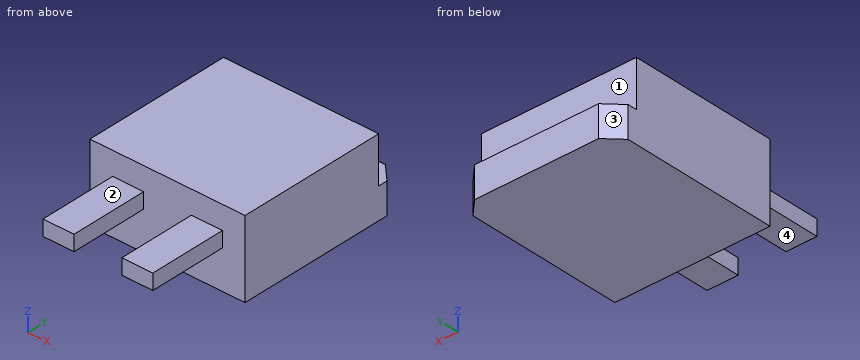
```python
from build123d import *

# Parameters (mm, degrees)
F0_W     = 10
F0_H     = 11.2
F1_DEPTH = 5
F2_W     = 10
F2_H     = 1.6
F3_DEPTH = 3
F4_SIZE  = 1
F5_W     = 2
F5_H     = 1
F6_DEPTH = 5


with BuildPart() as f1:
    # F0 (on Top) → F1 (new body)
    with BuildSketch(Plane.XY):
        with Locations((2.165886, -0.248423)):
            Rectangle(F0_W, F0_H)
    extrude(amount=F1_DEPTH)

    # F2 (on face) → F3 (cut)
    with BuildSketch(Plane.XY.offset(5)):
        with Locations((2.165886, 4.551577)):
            Rectangle(F2_W, F2_H)
    extrude(amount=-F3_DEPTH, mode=Mode.SUBTRACT)

    # F4
    f4_edges = [f1.edges().sort_by_distance(p)[0] for p in [
        (7.165886, 5.351577, 1),
        (-2.834114, 5.351577, 1),
    ]]
    chamfer(f4_edges, length=F4_SIZE)

    # F5 (on face) → F6 (join)
    with BuildSketch(Plane.XZ.offset(5.848423)):
        with Locations((-0.374114, 3)):
            Rectangle(F5_W, F5_H)
        with Locations((4.705886, 3)):
            Rectangle(F5_W, F5_H)
    extrude(amount=F6_DEPTH)


solid = f1.part
```
Check sheet for the modelled part. Datum: model origin and axes. Units: mm. Face numbers are marked on the shaded views. A direction names the side the tool comes from. Coordinates: 2 decimals unless noted, no trailing zeros. Write each loop counter-clockwise with the first axis right and the second up, starting at its lowest first coordinate (ties: lowest second). Pieces come first, ordered by that corner, then holes. Notation, with made-up numbers: (-31.75, -14) - (21.25, -14) arc R13 cw to (21.25, -10) - close; hole circle Ø10 at (76, 55). An arc over 180 degrees is marked (long way). One line per question, with ' | ' between items.
Item 1: Sectioned sample at B-B on z = 0.65. Record the boundary of the cut face in (x, y).
Determined:
outline: (-2.83, -5.85) - (7.17, -5.85) - (7.17, 4.35) - (6.17, 5.35) - (-1.83, 5.35) - (-2.83, 4.35) - close
Item 2: Access from +Z, -Z, +X, -X, +Y, -Y to the whole of each face (thin tool, end or side, straight path). Record for the marked faces 1, 2, 3 and 4.
Determined:
face 1: +Z, +X, -X, +Y | face 2: +Z, +X, -X, -Y | face 3: +Z, -Z, -X, +Y | face 4: -Z, +X, -X, -Y
Item 3: Sectioned sample at D-D on z = 2.2. Record the boundary of the cut face in (x, y).
Determined:
outline: (-2.83, -5.85) - (7.17, -5.85) - (7.17, 3.75) - (-2.83, 3.75) - close
Item 4: Thickness scan on line 1 (X direction, y = -6, z = 2.8); line 2 (Y direction, x = -1.25, z = 0.95); line 3 (Z direction, x = 4.5, y = -6). Record the ranges inside material, lowest first. Write a range as [from, to].
Determined:
line 1: x = [-1.37, 0.63], [3.71, 5.71] | line 2: y = [-5.85, 5.35] | line 3: z = [2.5, 3.5]
Item 5: Gauge pin test, flat ends, axial feed: P1, Ø0.9, axis at x = 1, z = 3, coming from the +Y side; P2, Ø0.5, axis at y = -9.5, z = 3, coming from the +X side; P3, Ø1, axis at x = 0, y = -8, coming from the -Z side. Record the tip position at first contact, or that the pin passes through.
Determined:
P1: stops at y = 3.75 | P2: stops at x = 5.71 | P3: stops at z = 2.5
Item 6: Sectioned sample at A-A on x = 5.25. Record the boundary of the cut face in (y, z).
Determined:
outline: (-10.85, 2.5) - (-5.85, 2.5) - (-5.85, 0) - (5.35, 0) - (5.35, 2) - (3.75, 2) - (3.75, 5) - (-5.85, 5) - (-5.85, 3.5) - (-10.85, 3.5) - close
Item 7: Sectioned sample at C-C on x = 1. Record the boundary of the cut face in (y, z).
Determined:
outline: (-5.85, 0) - (5.35, 0) - (5.35, 2) - (3.75, 2) - (3.75, 5) - (-5.85, 5) - close
